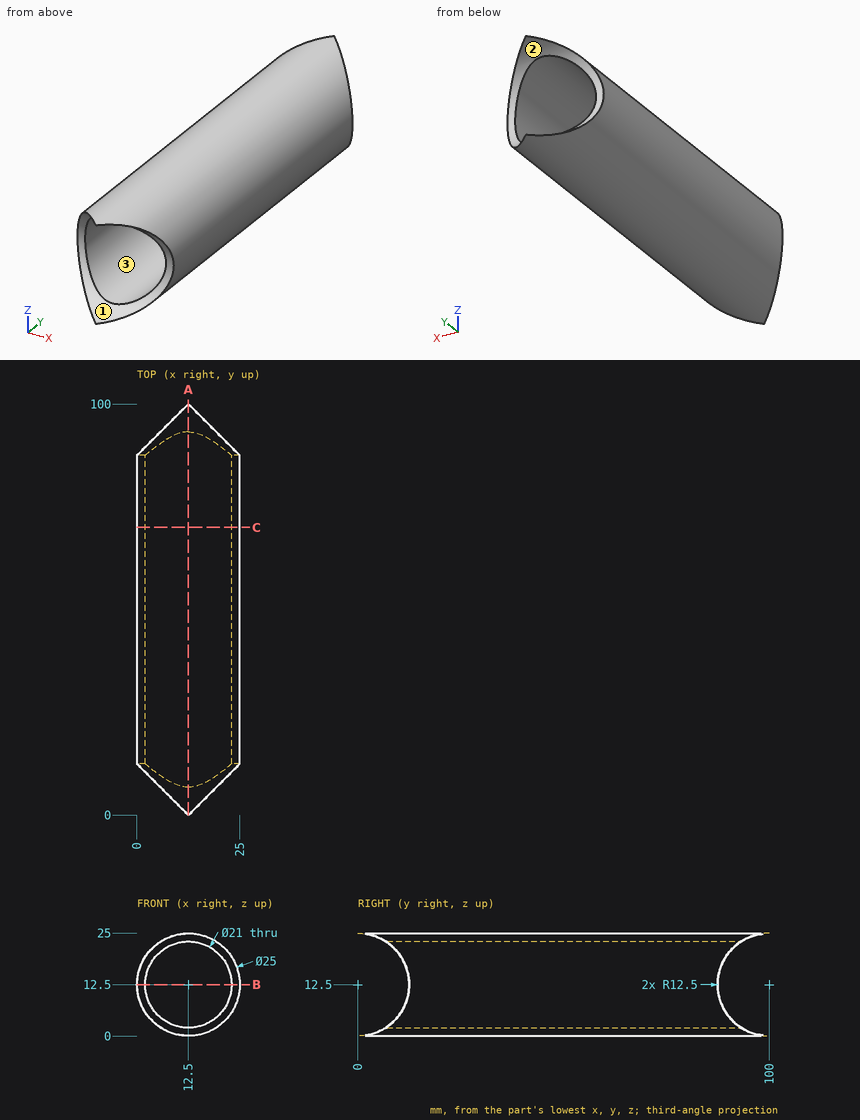
Job drawing, mm, ordinate dimensions from the low corner. One solid piece. Give positions to 0.01 mm unless a question says otherwise; leave off trailing zeros. Loops run counter-clockwise (first coordinate to the right, second up) from the corner with the lowest first, then second, coordinate; pieces in that order, holes last. Notation, with made-up numbers: (-6, 75) -> (-1, 75) arc R15 cw to (-1, 86) -> close; hole circle Ø4 at (81.25, 9). An arc over 180 degrees is marked (long way). Use a Markdown table: item, result. Add a question column.
(1) Slice it at C-C on y = 70. List the corners of the cut face in (x, z).
(2) Slice it at B-B on z = 12.5. List the corners of the cut face in (x, y), and give its area (3 significant figures).
(3) Drop flat-ended pins along their axis: pin 1 Ø8 at (y, z) = (80.5, 3.5) entering from -X; pin 2 Ø6 at (x, z) = (3, 10.5) entering from +Y; pin 3 Ø4 at (y, z) = (31.5, 7.5) entering from -X; pin 4 Ø10 at (y, z) = (80.5, 12) entering from +X. Give the stop position or say it passes through.
(4) Mould opens along Y. For the marked faces 1, 2 and 3 say: +Y half, -Y half, draft (parallel to the pull), parting line (faces both ways), or undercut.
(5) Slice it at A-A on x = 12.5. List the corners of the cut face in (y, z), and give its area (3 significant figures).
(6) Wall check: line 1 along Z through (x, y) = (12.75, 13.5); line 2 along Z through (x, y) = (6.25, 28); line 3 along X through (y, z) = (31.5, 9). Give the ranges that are in metal, low to high.
Filled sheet:
| question | item | result |
|---|---|---|
| 1 | outline | circle Ø25 at (12.5, 12.5); hole circle Ø21 at (12.5, 12.5) |
| 2 | outline | (0, 12.5) -> (2, 12.5) -> (2, 87.5) -> (0, 87.5) -> close; (23, 12.5) -> (25, 12.5) -> (25, 87.5) -> (23, 87.5) -> close |
| 2 | area | 300 mm2 |
| 3 | pin 1 | x = 1.04 |
| 3 | pin 2 | y = 88.54 |
| 3 | pin 3 | x = 0.37 |
| 3 | pin 4 | x = 25 |
| 4 | face 1 | -Y half |
| 4 | face 2 | +Y half |
| 4 | face 3 | draft |
| 5 | outline | (0, 0) -> (100, 0) arc R12.5 cw to (93.22, 2) -> (6.78, 2) arc R12.5 cw to start; (0, 25) arc R12.5 cw to (6.78, 23) -> (93.22, 23) arc R12.5 cw to (100, 25) -> close |
| 5 | area | 363 mm2 |
| 6 | line 1 | 0 to 2, 23 to 25 |
| 6 | line 2 | 1.67 to 4.06, 20.94 to 23.33 |
| 6 | line 3 | 0.5 to 2.6, 22.4 to 24.5 |
